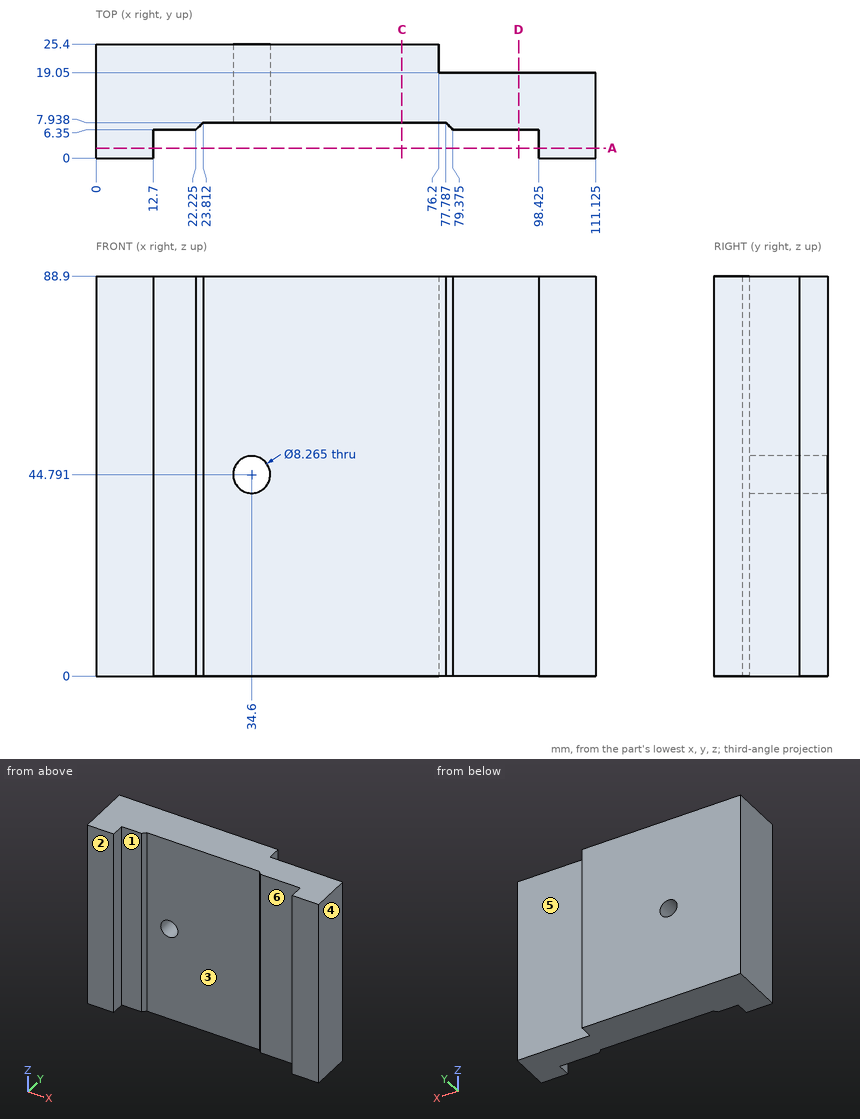
Print and shaded views of the part. All mm, measured from the part's lowest x, y and z. A direction names the side the tool comes from. Give positions to 0.01 mm unless a question says otherwise; leave off trailing zeros. Order: outer loops, then holes, each group sorted by start corner. A loop starts at its lowest first (then second) coordinate and runs counter-clockwise, first axis right, second up. Notation, with made-up numbers: (87.25, 58) -> (143.25, 58) arc R32 ccw to (143.25, 90) -> close; hole circle Ø1 at (1, -28.5). An arc over 180 degrees is marked (long way). Use CSV: the item, a comma, the result in double quotes.
1. Drill centre lines: line 1 along X through (y, z) = (3.5, 76.5) (1 decimal); line 2 along Y through (x, z) = (17.5, 19); line 3 along Y through (x, z) = (77.5, 32). Where is each one in solid material? Low to high. Write a range as from..to.
Outcome:
line 1,"0..12.7, 98.4..111.1"
line 2,"6.35..25.4"
line 3,"7.94..19.05"
2. 3-axis set-ups, long thin cutter, end or side, ignore diameter. For the marked faces 1 and 2: which of +Z, -Z, +X, -X, +Y, -Y reach the whole face in a straight line?
Outcome:
face 1,"+Z, -Z, -Y"
face 2,"+Z, -Z, +X, -X, -Y"
3. Mould opens along X. For the marked faces 3, 4, 5 and 6 say: +X half, -X half, draft (parallel to the pull), parting line (faces both ways), or undercut.
Outcome:
face 3,"undercut"
face 4,"+X half"
face 5,"draft"
face 6,"undercut"
4. Band-saw the part on D-D, the plane x = 94. Give the cut face in (y, z), then the cut area to 3 significant figures.
Outcome:
outline,"(6.35, 0) -> (19.05, 0) -> (19.05, 88.9) -> (6.35, 88.9) -> close"
area,"1,130 mm²"
5. Band-saw the part on C-C, the plane x = 68. Give the cut face in (y, z), then the cut area to 3 significant figures.
Outcome:
outline,"(7.94, 0) -> (25.4, 0) -> (25.4, 88.9) -> (7.94, 88.9) -> close"
area,"1,550 mm²"
6. Drop flat-ended pins along their axis: pin 1 (3 mm diameter, centred on x = 88, z = 77.5, fed in from +Y); pin 2 (5.5 mm diameter, centred on x = 90, z = 53.5, fed in from -Y); pin 3 (7 mm diameter, centred on y = 23.5, z = 64, fed in from +X); pin 4 (5 mm diameter, centred on x = 34.6, z = 44.79, fed in from -Y). Give the stop position or say it passes through.
Outcome:
pin 1,"y = 19.05"
pin 2,"y = 6.35"
pin 3,"x = 76.2"
pin 4,"through"
7. Band-saw the part on A-A, the plane y = 2.25. Give the cut face in (x, z) (1 decimal).
Outcome:
outline,"(0, 0) -> (12.7, 0) -> (12.7, 88.9) -> (0, 88.9) -> close; (98.4, 0) -> (111.1, 0) -> (111.1, 88.9) -> (98.4, 88.9) -> close"
